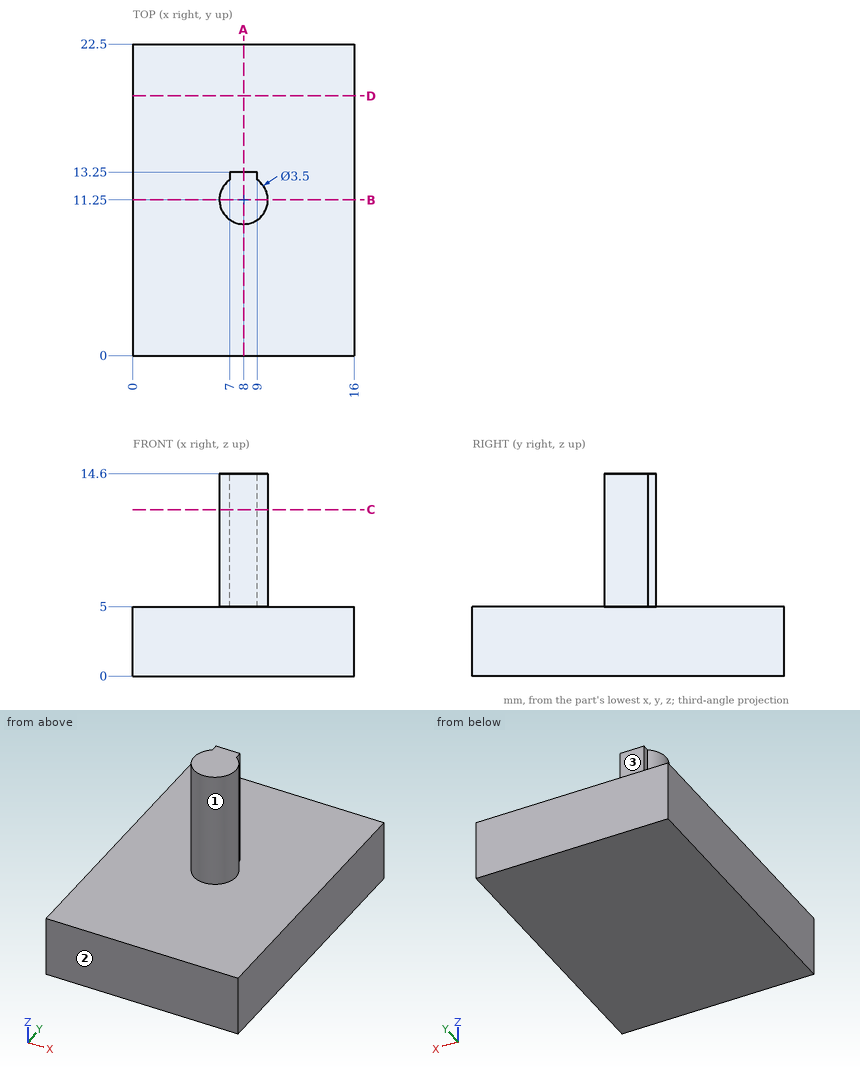
Study the drawing (mm; zero at the part's minimum x, y, z) and answer. A direction names the side the tool comes from. Round coordinates to 2 decimals unless told otherwise and drop trailing zeros. Order: outer loops, then holes, each group sorted by start corner. A loop starts at its lowest first (then second) coordinate and runs counter-clockwise, first axis right, second up. Notation, with made-up numbers: (-19.75, 38) -> (-2.75, 38) arc R23 ccw to (-2.75, 67) -> close; hole circle Ø11 at (34, -27.5). An arc over 180 degrees is marked (long way). Answer as CSV lines item,"result". Start each with the question number.
(1) The part is cut by section A-A (x = 8). Determine the outline of the cut face in (y, z).
(2) The part is cut by section C-C (z = 12). Determine the outline of the cut face in (x, y).
(3) Find the intervals of material crossed by probe 1 along Z at (x, y) = (6.75, 6); probe 2 along X at (y, z) = (10, 13.5); probe 3 along Y at (x, z) = (9.25, 5.5), in increasing order. Write a range as from..to.
(4) Flat-ended cylindrical pins translate along their axes: pin 1 Ø6 at (y, z) = (10.5, 8.5) entering from -X; pin 2 Ø5 at (x, y) = (12, 7) entering from +Z; pin 3 Ø2 at (x, z) = (8, 12) entering from +Y. Find the tip coordinate at first contact, or state that the pin passes through.
(5) The part is cut by section B-B (y = 11.25). Determine the outline of the cut face in (x, z), then the cut area to 3 significant figures.
(6) A tool of negligible diameter and unlimited length cuts with its end or side. For the marked faces 1, 2 and 3, from which of +Z, -Z, +X, -X, +Y, -Y can it reach the whole face along a straight path? Write none if from no direction.
(7) The part is cut by section D-D (y = 18.75). Determine the outline of the cut face in (x, z), then the cut area to 3 significant figures.
Evaluation:
1,outline,"(0, 0) -> (22.5, 0) -> (22.5, 5) -> (13.25, 5) -> (13.25, 14.6) -> (9.5, 14.6) -> (9.5, 5) -> (0, 5) -> close"
2,outline,"(7, 12.69) arc R1.75 ccw (long way) to (9, 12.69) -> (9, 13.25) -> (7, 13.25) -> close"
3,probe 1,"0..5"
3,probe 2,"6.78..9.22"
3,probe 3,"10.03..12.47"
4,pin 1,"x = 6.25"
4,pin 2,"z = 5"
4,pin 3,"y = 13.25"
5,outline,"(0, 0) -> (16, 0) -> (16, 5) -> (9.75, 5) -> (9.75, 14.6) -> (6.25, 14.6) -> (6.25, 5) -> (0, 5) -> close"
5,area,"114 mm²"
6,face 1,"+Z"
6,face 2,"+Z, -Z, +X, -X, -Y"
6,face 3,"+Z, +X, -X, +Y"
7,outline,"(0, 0) -> (16, 0) -> (16, 5) -> (0, 5) -> close"
7,area,"80.0 mm²"
